```python
from build123d import *

# Parameters (mm, degrees)
SKETCH1_R           = 5
BOSS_EXTRUDE1_DEPTH = 5.5
SKETCH2_R           = 1.35
CUT_EXTRUDE1_DEPTH  = 10


with BuildPart() as part:
    # Sketch1 → Boss-Extrude1 (new body)
    with BuildSketch(Plane(origin=(0, 0, 0), x_dir=(1, 0, 0), z_dir=(0, 1, 0))):
        with BuildLine():
            Line((-10, 0), (-8.5, 14))
            ThreePointArc((-8.5, 14), (0, 22.5), (8.5, 14))
            Line((8.5, 14), (10, 0))
            Line((10, 0), (-10, 0))
        make_face()
        with Locations(Location((0, 14, 0), (0, 0, 270))):
            Circle(SKETCH1_R, mode=Mode.SUBTRACT)
    extrude(amount=BOSS_EXTRUDE1_DEPTH)

    # Sketch2 → Cut-Extrude1 (cut)
    with BuildSketch(Plane.XY):
        with Locations((-7, 2.75)):
            Circle(SKETCH2_R)
        with Locations(Location((7, 2.75, 0), (0, 0, 180))):
            Circle(SKETCH2_R)
    extrude(amount=-CUT_EXTRUDE1_DEPTH, mode=Mode.SUBTRACT)


solid = part.part
```
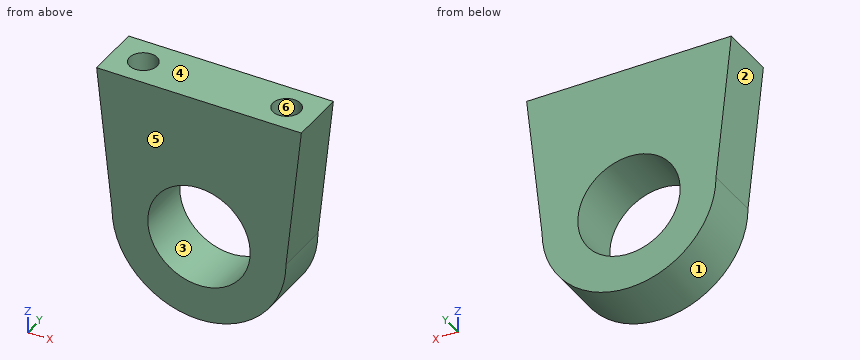
Model file for the job. Use its own axes, mm. Face numbers are marked on the shaded views. A direction names the side the tool comes from. Coordinates: 2 decimals unless noted, no trailing zeros. Loops run counter-clockwise (first coordinate to the right, second up) from the corner with the lowest first, then second, coordinate; pieces in that order, holes last. Notation, with made-up numbers: (7.5, 17.25) - (23.5, 17.25) arc R10 cw to (23.5, 33.25) - close; hole circle Ø6 at (64, -30). An arc over 180 degrees is marked (long way). Answer as a JSON object with one key per item and string values. Group by question number.
(1) Cut at A-A (y = 2.75). Give the cut face in (x, z).
(2) Flat gauge pins, fed straight in: pin 1 (3 mm diameter, centred on x = 7.5, y = 3, fed in from +Z); pin 2 (2 mm diameter, centred on x = -7, y = 2.75, fed in from -Z); pin 3 (2 mm diameter, centred on x = -6.5, y = 4.5, fed in from -Z). Where does each tip first touch, or does it go through?
(3) Cut at D-D (x = 8). Give the cut face in (y, z).
(4) Probe line 1 along X through (y, z) = (3.9, -14); line 2 along Y through (x, z) = (-7, -7.25); line 3 along X through (y, z) = (3.35, -9.5). List the from-to ranges inside material, lowest first.
(5) Tool access for the marked faces 5 and 6: list every direction of +Z, -Z, +X, -X, +Y, -Y with a clear straight run to the whole face (end or side of a thin tool).
(6) Two-plate mould, pull along X, no slides. Class the marked faces 1, 2, 3 and 4: released by +X, released by -X, zero draft, split by the parting line, or undercut.
(7) Cut at C-C (z = -17.25). Give the cut face in (x, y), then the cut area to 3 significant figures.
(8) Cut at B-B (x = 0). Give the cut face in (y, z).
Geometry says:
{
 "1": {"outline": "(-10, 0) - (-8.5, -14) arc R8.5 ccw to (8.5, -14) - (10, 0) - (8.35, 0) - (8.35, -10) - (5.65, -10) - (5.65, 0) - (-5.65, 0) - (-5.65, -10) - (-8.35, -10) - (-8.35, 0) - close; hole circle Ø10 at (0, -14)"},
 "2": {"pin 1": "stops at z = 0", "pin 2": "stops at z = -20.02", "pin 3": "stops at z = -20.48"},
 "3": {"outline": "(0, -16.87) - (5.5, -16.87) - (5.5, 0) - (3.66, 0) - (3.66, -10) - (1.84, -10) - (1.84, 0) - (0, 0) - close"},
 "4": {"line 1": "x = -8.5 to -5, 5 to 8.5", "line 2": "y = 0 to 1.4, 4.1 to 5.5", "line 3": "x = -8.98 to -8.21, -5.79 to -2.18, 2.18 to 5.79, 8.21 to 8.98"},
 "5": {"face 5": "+Z, -Z, +X, -X, -Y", "face 6": "+Z"},
 "6": {"face 1": "split by the parting line", "face 2": "released by -X", "face 3": "undercut", "face 4": "zero draft"},
 "7": {"outline": "(-7.85, 0) - (-3.8, 0) - (-3.8, 5.5) - (-7.85, 5.5) - close; (3.8, 0) - (7.85, 0) - (7.85, 5.5) - (3.8, 5.5) - close", "area": "44.6 mm^2"},
 "8": {"outline": "(0, -22.5) - (5.5, -22.5) - (5.5, -19) - (0, -19) - close; (0, -9) - (5.5, -9) - (5.5, 0) - (0, 0) - close"}
}
